For this review, take the finished solid that the model builds, in its own axes (mm). A direction names the side the tool comes from. Round coordinates to 2 decimals unless told otherwise and drop trailing zeros. Order: outer loops, then holes, each group sorted by start corner. A loop starts at its lowest first (then second) coordinate and runs counter-clockwise, first axis right, second up. Notation, with made-up numbers: (-3.5, 21) - (10.5, 21) arc R21 ccw to (10.5, 41) - close; hole circle Ø9 at (10.5, 86.5). An arc over 180 degrees is marked (long way). One line per question, with ' | ' between items.
```python
from build123d import *

# Parameters (mm, degrees)
SKETCH1_W                                           = 92.56
SKETCH1_H                                           = 46
BOSS_EXTRUDE1_DEPTH                                 = 6
SKETCH2_W                                           = 7
SKETCH2_H                                           = 46
BOSS_EXTRUDE2_DEPTH                                 = 54
SKETCH3_R                                           = 16
CUT_EXTRUDE1_DEPTH                                  = 120.512985069
SKETCH4_R                                           = 16
CUT_EXTRUDE2_DEPTH                                  = 117.616266447
F_4_2_4_2_DIAMETER_HOLE1_D                          = 4.2
F_4_2_4_2_DIAMETER_HOLE2_D                          = 4.2
CHAMFER1_SIZE                                       = 3.5
CHAMFER2_SIZE                                       = 6
BOSS_EXTRUDE3_DEPTH                                 = 46
FILLET1_R                                           = 2.5
CHAMFER3_SIZE                                       = 2.5
FILLET2_R                                           = 2.5
CSK_FOR_M3_COUNTERSUNK_FLAT_HEAD_SCREW1_D           = 3.2
CSK_FOR_M3_COUNTERSUNK_FLAT_HEAD_SCREW1_DEPTH       = 30
CSK_FOR_M3_COUNTERSUNK_FLAT_HEAD_SCREW1_CSINK_D     = 6.3
CSK_FOR_M3_COUNTERSUNK_FLAT_HEAD_SCREW1_CSINK_ANGLE = 90
CSK_FOR_M3_COUNTERSUNK_FLAT_HEAD_SCREW1_TIP         = 0.96137699
CSK_FOR_M3_COUNTERSUNK_FLAT_HEAD_SCREW2_D           = 3.6
CSK_FOR_M3_COUNTERSUNK_FLAT_HEAD_SCREW2_DEPTH       = 30
CSK_FOR_M3_COUNTERSUNK_FLAT_HEAD_SCREW2_CSINK_D     = 6.3
CSK_FOR_M3_COUNTERSUNK_FLAT_HEAD_SCREW2_CSINK_ANGLE = 90
CSK_FOR_M3_COUNTERSUNK_FLAT_HEAD_SCREW2_TIP         = 1.081549114
SKETCH18_W                                          = 2.5
SKETCH18_H                                          = 5.65
CUT_EXTRUDE4_DEPTH                                  = 121.623188484


with BuildPart() as part:
    # Sketch1 → Boss-Extrude1 (new body)
    with BuildSketch(Plane(origin=(0, 0, 0), x_dir=(1, 0, 0), z_dir=(0, 1, 0))):
        with Locations((46.28, 23)):
            Rectangle(SKETCH1_W, SKETCH1_H)
    extrude(amount=BOSS_EXTRUDE1_DEPTH)

    # Sketch2 → Boss-Extrude2 (add)
    with BuildSketch(Plane(origin=(0, 6, 0), x_dir=(1, 0, 0), z_dir=(0, 1, 0))):
        with Locations((89.06, 23)):
            Rectangle(SKETCH2_W, SKETCH2_H)
        with Locations((3.5, 23)):
            Rectangle(SKETCH2_W, SKETCH2_H)
    extrude(amount=BOSS_EXTRUDE2_DEPTH)

    # Sketch3 → Cut-Extrude1 (cut, through all)
    with BuildSketch(Plane(origin=(92.56, 0, 0), x_dir=(0, 0, -1), z_dir=(1, 0, 0))):
        with Locations((23, 37)):
            Circle(SKETCH3_R)
    extrude(amount=-CUT_EXTRUDE1_DEPTH, mode=Mode.SUBTRACT)

    # Sketch4 → Cut-Extrude2 (cut, through all)
    with BuildSketch(Plane(origin=(0, 6, 0), x_dir=(1, 0, 0), z_dir=(0, 1, 0))):
        with Locations(Location((46.28, 23, 0), (0, 0, 270))):
            Circle(SKETCH4_R)
    extrude(amount=-CUT_EXTRUDE2_DEPTH, mode=Mode.SUBTRACT)

    # Ø4.2 (4.2) Diameter Hole1 (through all)
    with Locations(Plane(origin=(0, 0, 0), x_dir=(-1, 0, 0), z_dir=(0, -1, 0))):
        with Locations((-63.165621688, 39.642079068), (-29.637920932, 39.885621688), (-29.394378312, 6.357920932), (-62.922079068, 6.114378312)):
            Hole(F_4_2_4_2_DIAMETER_HOLE1_D / 2)

    # Ø4.2 (4.2) Diameter Hole2 (through all)
    with Locations(Plane.ZY):
        with Locations((-39.885621688, 53.642079068), (-6.357920932, 53.885621688), (-6.114378312, 20.357920932), (-39.642079068, 20.114378312)):
            Hole(F_4_2_4_2_DIAMETER_HOLE2_D / 2)

    # Chamfer1
    chamfer1_edges = [part.edges().sort_by_distance(p)[0] for p in [
        (89.06, 60, -46),
        (89.06, 60, 0),
        (3.5, 60, 0),
        (3.5, 60, -46),
    ]]
    chamfer(chamfer1_edges, length=CHAMFER1_SIZE)

    # Chamfer2
    chamfer2_edges = [part.edges().sort_by_distance(p)[0] for p in [
        (85.56, 6, -23),
        (7, 6, -23),
    ]]
    chamfer(chamfer2_edges, length=CHAMFER2_SIZE)

    # Sketch10 → Boss-Extrude3 (add)
    with BuildSketch(Plane(origin=(0, 0, -46), x_dir=(-1, 0, 0), z_dir=(0, 0, -1))):
        Polygon((0, 11), (5, 11), (5, -5), (-11, -5), (-11, 0), (0, 0), align=None)
        Polygon((-81.56, 0), (-92.56, 0), (-92.56, 11), (-97.56, 11), (-97.56, -5), (-81.56, -5), align=None)
    extrude(amount=-BOSS_EXTRUDE3_DEPTH)

    # Fillet1
    fillet1_edges = [part.edges().sort_by_distance(p)[0] for p in [
        (-5, 11, -23),
        (11, -5, -23),
        (81.56, -5, -23),
        (97.56, 11, -23),
    ]]
    fillet(fillet1_edges, radius=FILLET1_R)

    # Chamfer3
    chamfer3_edges = [part.edges().sort_by_distance(p)[0] for p in [
        (92.56, 11, -23),
        (81.56, 0, -23),
        (11, 0, -23),
        (0, 11, -23),
    ]]
    chamfer(chamfer3_edges, length=CHAMFER3_SIZE - 0.0001)  # a hair under: the kernel refuses the full size

    # Fillet2
    fillet2_edges = [part.edges().sort_by_distance(p)[0] for p in [
        (-5, -5, -23),
        (97.56, -5, -23),
    ]]
    fillet(fillet2_edges, radius=FILLET2_R)

    # CSK for M3 Countersunk Flat Head Screw1
    with Locations(Plane.ZY.offset(5)):
        with Locations((-11, 3), (-23, 3), (-35, 3)):
            CounterSinkHole(CSK_FOR_M3_COUNTERSUNK_FLAT_HEAD_SCREW1_D / 2, CSK_FOR_M3_COUNTERSUNK_FLAT_HEAD_SCREW1_CSINK_D / 2, depth=CSK_FOR_M3_COUNTERSUNK_FLAT_HEAD_SCREW1_DEPTH, counter_sink_angle=CSK_FOR_M3_COUNTERSUNK_FLAT_HEAD_SCREW1_CSINK_ANGLE)
            with Locations((0, 0, -(CSK_FOR_M3_COUNTERSUNK_FLAT_HEAD_SCREW1_DEPTH + CSK_FOR_M3_COUNTERSUNK_FLAT_HEAD_SCREW1_TIP / 2))):  # 118° drill point
                Cone(0, CSK_FOR_M3_COUNTERSUNK_FLAT_HEAD_SCREW1_D / 2, CSK_FOR_M3_COUNTERSUNK_FLAT_HEAD_SCREW1_TIP, mode=Mode.SUBTRACT)

    # CSK for M3 Countersunk Flat Head Screw2
    with Locations(Plane(origin=(97.56, 0, 0), x_dir=(0, 0, -1), z_dir=(1, 0, 0))):
        with Locations((11, 3), (23, 3), (35, 3)):
            CounterSinkHole(CSK_FOR_M3_COUNTERSUNK_FLAT_HEAD_SCREW2_D / 2, CSK_FOR_M3_COUNTERSUNK_FLAT_HEAD_SCREW2_CSINK_D / 2, depth=CSK_FOR_M3_COUNTERSUNK_FLAT_HEAD_SCREW2_DEPTH, counter_sink_angle=CSK_FOR_M3_COUNTERSUNK_FLAT_HEAD_SCREW2_CSINK_ANGLE)
            with Locations((0, 0, -(CSK_FOR_M3_COUNTERSUNK_FLAT_HEAD_SCREW2_DEPTH + CSK_FOR_M3_COUNTERSUNK_FLAT_HEAD_SCREW2_TIP / 2))):  # 118° drill point
                Cone(0, CSK_FOR_M3_COUNTERSUNK_FLAT_HEAD_SCREW2_D / 2, CSK_FOR_M3_COUNTERSUNK_FLAT_HEAD_SCREW2_TIP, mode=Mode.SUBTRACT)

    # Sketch18 → Cut-Extrude4 (cut, through all)
    with BuildSketch(Plane(origin=(0, 6, 0), x_dir=(1, 0, 0), z_dir=(0, 1, 0))):
        with Locations((22, 23)):
            Rectangle(SKETCH18_W, SKETCH18_H)
        with Locations((22, 35)):
            Rectangle(SKETCH18_W, SKETCH18_H)
        with Locations((22, 11)):
            Rectangle(SKETCH18_W, SKETCH18_H)
    cut_extrude4 = extrude(amount=-CUT_EXTRUDE4_DEPTH, mode=Mode.SUBTRACT)

    # Mirror1: Cut-Extrude4 across plane
    add(cut_extrude4.mirror(Plane.ZY.offset(-46.28)), mode=Mode.SUBTRACT)

    # SurfaceCut1
    split(bisect_by=Plane(origin=(7, 0, 0), x_dir=(0, 0, -1), z_dir=(1, 0, 0)), keep=Keep.TOP)

    # SurfaceCut2
    split(bisect_by=Plane.ZY.offset(-85.56), keep=Keep.TOP)


solid = part.part
```
(1) We need section A-A on y = 7.25. State the section outline as (x, z) points, plus the area to 3 significant figures.
Output values:
outline: (7, -46) - (11.75, -46) - (11.75, 0) - (7, 0) - close; (80.81, -46) - (85.56, -46) - (85.56, 0) - (80.81, 0) - close | area: 437 mm^2
(2) Insertion check: pin 1 (2.5 mm diameter, centred on y = 3, z = -11, fed in from +X); pin 2 (2 mm diameter, centred on x = 19, z = -38, fed in from -Y); pin 3 (10 mm diameter, centred on x = 57.5, z = -14.5, fed in from +Y). Each pin has a flat end and moves straight along its axis. Give the tip position at first contact, or say it passes through.
Output values:
pin 1: x = 67.23 | pin 2: y = 0 | pin 3: y = 6
(3) We need section C-C on x = 46.28. State the section outline as (y, z) points.
Output values:
outline: (0, -46) - (6, -46) - (6, -39) - (0, -39) - close; (0, -7) - (6, -7) - (6, 0) - (0, 0) - close
(4) For probe 1 along Z at (x, y) = (23.8, 3); probe 2 along Z at (x, y) = (68.6, 3); probe 3 along X at (y, z) = (-1.75, -12), list the stretches that pass through material, from the lowest coordinate up. Write a range as [from, to].
Output values:
probe 1: [-46, -36.6], [-33.4, -24.6], [-21.4, -12.6], [-9.4, 0] | probe 2: [-46, -36.8], [-33.2, -24.8], [-21.2, -12.8], [-9.2, 0] | probe 3: [7, 11.75], [80.81, 85.56]
(5) For faces 5 (the flat face through (23.25, 4.4, -24.2)), 6 (the flat face through (31, 6, -28.4)), 7 (the cylindrical face through (78.589, 3.541, -33.283)), list the 3-axis set-ups (+Z, -Z, +X, -X, +Y, -Y) from which the entire face can be reached by the end or side of a thin tool; tool diameter is ignored.
Output values:
face 5: +Y, -Y | face 6: +Z, -Z, +Y | face 7: +X
(6) Mouldability with a two-part tool opening along Z and no side actions: class faces 1 (the flat face through (8, -5, -23)), 2 (the flat face through (46, 4, -46)), 3 (the flat face through (71, 3, -37.825)), 4 (the flat face through (20.75, 4.4, -12.2)) as released by +Z, released by -Z, zero draft, split by the parting line, or undercut.
Output values:
face 1: zero draft | face 2: released by -Z | face 3: undercut | face 4: undercut
(7) We need section B-B on x = 20. State the section outline as (y, z) points, plus the area to 3 significant figures.
Output values:
outline: (0, -46) - (6, -46) - (6, 0) - (0, 0) - close; hole circle Ø3.2 at (3, -35); hole circle Ø3.2 at (3, -23); hole circle Ø3.2 at (3, -11) | area: 252 mm^2
